Here's how the part is built. I have some questions about the finished solid (model axes, mm). A direction names the side the tool comes from. Coordinates: 2 decimals unless noted, no trailing zeros. Loops run counter-clockwise (first coordinate to the right, second up) from the corner with the lowest first, then second, coordinate; pieces in that order, holes last. Notation, with made-up numbers: M 5.25,-30 L 10.25,-30 A30 ccw 10.25,5 Z; hole C -4.75,11 d6. An arc over 180 degrees is marked long. Use one line per item in the form item = value. Start each with the question number.
(1) Imagine slicing it at B-B, the plane y = -17.5. Please give me the cut outline in (x, z), and give its area (3 significant figures).
(2) On a 3-axis mill with a long thin cutter (end or side, diameter ignored), from which of +Z, -Z, +X, -X, +Y, -Y can I reach the whole of each face in a straight line? I mean faces 1 (the flat face through (9.329, -13, -61)), 2 (the flat face through (-6.824, -22.824, 1.791)), 3 (the flat face through (-14, -13, -46.523)). Say none if no direction works.
(3) Please list where these lines run through material, in increasing order: L1, parallel to Z at x = 16, y = -7; L2, parallel to X at y = -13, z = 27; L3, parallel to Y at x = 6, z = 38.5.
(4) Will these pins go through, and if not, where does the flat tip stop? P1, Ø12, axis at y = -10.5, z = 6, coming from the +X side; P2, Ø10, axis at x = -10.5, y = -22.5, coming from the +Z side; P3, Ø12, axis at y = -14.5, z = 4.5, coming from the -X side; P4, Ø10, axis at x = 13, y = -15, coming from the -Z side.
(5) Imagine slicing it at C-C, the plane x = 11. Please give me the cut outline in (y, z).
(6) Imagine slicing it at D-D, the plane x = -6.5. Please give me the cut outline in (y, z), and give its area (3 significant figures).
(7) Imagine slicing it at A-A, the plane z = -7. Please give me the cut outline in (x, y), and give its area (3 significant figures).
```python
from build123d import *

# Parameters (mm, degrees)
F0_W        = 9.0893283486
F0_H        = 21.5273555368
F0_W_2      = 9.3285199255
F0_H_2      = 29.4207185507
F1_DEPTH    = 25.4
F2_R        = 9.5587418967
F3_DEPTH    = 25.4
F4_C1_SIZE  = 5.08
F4_C2_SIZE  = 5.08
F4_C3_SIZE  = 5.08
F4_C4_SIZE  = 5.08
F4_C5_SIZE  = 5.08
F4_C6_SIZE  = 5.0799
F4_C7_SIZE  = 5.08
F4_C8_SIZE  = 5.08
F4_C9_SIZE  = 5.08
F4_C10_SIZE = 5.08
F4_C11_SIZE = 5.08
F4_C12_SIZE = 5.08
F5_C1_SIZE  = 5.08
F5_C2_SIZE  = 5.08
F5_C3_SIZE  = 5.08
F5_C4_SIZE  = 5.08
F5_C5_SIZE  = 5.08
F5_C6_SIZE  = 5.08
F5_C7_SIZE  = 5.08
F5_C8_SIZE  = 5.08
F5_C9_SIZE  = 5.08
F5_C10_SIZE = 5.08
F5_C11_SIZE = 5.0799
F5_C12_SIZE = 5.08


# Not quite as in the source:
# - a fillet or chamfer is up to 0.001 mm smaller than in the source, because OpenCascade refuses the exact size


with BuildPart() as f1:
    # F0 (on Front) → F1 (new body)
    with BuildSketch(Plane.XZ):
        with Locations((-13.8731840998, -35.7593270019)):
            Rectangle(F0_W, F0_H)
        Polygon((-9.3285199255, -24.9956492335), (-9.3285199255, -46.5230047703), (0, -46.5230047703), (9.3285199255, -46.5230047703), (9.3285199255, -24.9956492335), (9.3285199255, 34.5633625984), (9.3285199255, 71.3990554214), (6.6973981448, 68.2895556092), (-9.3285199255, 34.5633625984), align=None)
        with Locations((13.8731840998, -35.7593270019)):
            Rectangle(F0_W, F0_H)
        with Locations((-4.6642599627, -61.2333640456)):
            Rectangle(F0_W_2, F0_H_2)
        with Locations((4.6642599627, -61.2333640456)):
            Rectangle(F0_W_2, F0_H_2)
    extrude(amount=F1_DEPTH)

    # F2 (on Front) → F3 (join)
    with BuildSketch(Plane.XZ):
        with Locations((0, -37.1944867074)):
            Circle(F2_R)
    extrude(amount=F3_DEPTH)

    # F4: chamfer of 5.08 on 13 edges, made by hand

    # F4_c1
    f4_c1_edges = [f1.edges().sort_by_distance(p)[0] for p in [
        (-13.8731840998, 0, -46.5230047703),
    ]]
    chamfer(f4_c1_edges, length=F4_C1_SIZE)

    # F4_c2
    f4_c2_edges = [f1.edges().sort_by_distance(p)[0] for p in [
        (-18.4178482741, 0, -33.2193270019),
    ]]
    chamfer(f4_c2_edges, length=F4_C2_SIZE)

    # F4_c3
    f4_c3_edges = [f1.edges().sort_by_distance(p)[0] for p in [
        (-9.3285199255, 0, -61.2333640456),
    ]]
    chamfer(f4_c3_edges, length=F4_C3_SIZE)

    # F4_c4
    f4_c4_edges = [f1.edges().sort_by_distance(p)[0] for p in [
        (2.54, 0, -75.943723321),
    ]]
    chamfer(f4_c4_edges, length=F4_C4_SIZE)

    # F4_c5
    f4_c5_edges = [f1.edges().sort_by_distance(p)[0] for p in [
        (9.3285199255, 0, -58.6933640456),
    ]]
    chamfer(f4_c5_edges, length=F4_C5_SIZE)

    # F4_c6 (size 5.08 in the source; OpenCascade refuses exactly that, so slightly less here)
    f4_c6_edges = [f1.edges().sort_by_distance(p)[0] for p in [
        (13.8731840998, 0, -46.5230047703),
    ]]
    chamfer(f4_c6_edges, length=F4_C6_SIZE)

    # F4_c7
    f4_c7_edges = [f1.edges().sort_by_distance(p)[0] for p in [
        (18.4178482741, 0, -33.2193770019),
    ]]
    chamfer(f4_c7_edges, length=F4_C7_SIZE)

    # F4_c8
    f4_c8_edges = [f1.edges().sort_by_distance(p)[0] for p in [
        (11.3331840998, 0, -24.9956492335),
    ]]
    chamfer(f4_c8_edges, length=F4_C8_SIZE)

    # F4_c9
    f4_c9_edges = [f1.edges().sort_by_distance(p)[0] for p in [
        (9.3285199255, 0, 23.2017030939),
    ]]
    chamfer(f4_c9_edges, length=F4_C9_SIZE)

    # F4_c10
    f4_c10_edges = [f1.edges().sort_by_distance(p)[0] for p in [
        (-2.54, 0, 48.8496538587),
    ]]
    chamfer(f4_c10_edges, length=F4_C10_SIZE)

    # F4_c11
    f4_c11_edges = [f1.edges().sort_by_distance(p)[0] for p in [
        (-9.3285199255, 0, -1.1343040268),
    ]]
    chamfer(f4_c11_edges, length=F4_C11_SIZE)

    # F4_c12
    f4_c12_edges = [f1.edges().sort_by_distance(p)[0] for p in [
        (-11.3331840998, 0, -24.9956492335),
    ]]
    chamfer(f4_c12_edges, length=F4_C12_SIZE)

    # F5: chamfer of 5.08 on 13 edges, made by hand

    # F5_c1
    f5_c1_edges = [f1.edges().sort_by_distance(p)[0] for p in [
        (-18.4178482741, -25.4, -35.7593270019),
    ]]
    chamfer(f5_c1_edges, length=F5_C1_SIZE)

    # F5_c2
    f5_c2_edges = [f1.edges().sort_by_distance(p)[0] for p in [
        (-11.3331840998, -25.4, -24.9956492335),
    ]]
    chamfer(f5_c2_edges, length=F5_C2_SIZE)

    # F5_c3
    f5_c3_edges = [f1.edges().sort_by_distance(p)[0] for p in [
        (-11.3331840998, -25.4, -46.5230047703),
    ]]
    chamfer(f5_c3_edges, length=F5_C3_SIZE)

    # F5_c4
    f5_c4_edges = [f1.edges().sort_by_distance(p)[0] for p in [
        (-9.3285199255, -25.4, 4.7838566825),
    ]]
    chamfer(f5_c4_edges, length=F5_C4_SIZE)

    # F5_c5
    f5_c5_edges = [f1.edges().sort_by_distance(p)[0] for p in [
        (-9.3285199255, -25.4, -61.2333640456),
    ]]
    chamfer(f5_c5_edges, length=F5_C5_SIZE)

    # F5_c6
    f5_c6_edges = [f1.edges().sort_by_distance(p)[0] for p in [
        (1.2244391096, -25.4, 56.7718333827),
    ]]
    chamfer(f5_c6_edges, length=F5_C6_SIZE)

    # F5_c7
    f5_c7_edges = [f1.edges().sort_by_distance(p)[0] for p in [
        (2.54, -25.4, -75.943723321),
    ]]
    chamfer(f5_c7_edges, length=F5_C7_SIZE)

    # F5_c8
    f5_c8_edges = [f1.edges().sort_by_distance(p)[0] for p in [
        (9.3285199255, -25.4, 18.4973615123),
    ]]
    chamfer(f5_c8_edges, length=F5_C8_SIZE)

    # F5_c9
    f5_c9_edges = [f1.edges().sort_by_distance(p)[0] for p in [
        (13.8731840998, -25.4, -46.5230047703),
    ]]
    chamfer(f5_c9_edges, length=F5_C9_SIZE)

    # F5_c10
    f5_c10_edges = [f1.edges().sort_by_distance(p)[0] for p in [
        (9.3285199255, -25.4, -58.6933640456),
    ]]
    chamfer(f5_c10_edges, length=F5_C10_SIZE)

    # F5_c11 (size 5.08 in the source; OpenCascade refuses exactly that, so slightly less here)
    f5_c11_edges = [f1.edges().sort_by_distance(p)[0] for p in [
        (13.8731840998, -25.4, -24.9956492335),
    ]]
    chamfer(f5_c11_edges, length=F5_C11_SIZE)

    # F5_c12
    f5_c12_edges = [f1.edges().sort_by_distance(p)[0] for p in [
        (18.4178482741, -25.4, -35.7592770019),
    ]]
    chamfer(f5_c12_edges, length=F5_C12_SIZE)


solid = f1.part
```
Answer:
q1.outline = M -18.42,-46.52 L -9.33,-46.52 L -9.33,-75.94 L 9.33,-75.94 L 9.33,-46.52 L 18.42,-46.52 L 18.42,-25 L 9.33,-25 L 9.33,71.4 L 6.7,68.29 L -9.33,34.56 L -9.33,-25 L -18.42,-25 Z
q1.area = 2,820 mm²
q2.face_1 = -Z, +X, +Y, -Y
q2.face_2 = +Z, -X, -Y
q2.face_3 = -Z, -X, +Y, -Y
q3.L1 = -46.52 to -25
q3.L2 = -9.33 to 9.33
q3.L3 = -23.65 to -1.75
q4.P1 = 9.33
q4.P2 = 41.57
q4.P3 = -9.33
q4.P4 = -75.94
q5.outline = M -25.4,-41.44 L -20.32,-46.52 L -5.08,-46.52 L 0,-41.44 L 0,-30.08 L -5.08,-25 L -20.32,-25 L -25.4,-30.08 Z
q6.outline = M -25.4,-41.44 L -23.15,-43.69 L -23.15,-73.12 L -20.32,-75.94 L -5.08,-75.94 L -2.25,-73.12 L -2.25,-43.69 L 0,-41.44 L 0,-30.08 L -2.25,-27.82 L -2.25,33.93 L -5.08,40.52 L -20.32,40.52 L -23.15,33.93 L -23.15,-27.82 L -25.4,-30.08 Z
q6.area = 2,470 mm²
q7.outline = M -9.33,-20.32 L -4.25,-25.4 L 4.25,-25.4 L 9.33,-20.32 L 9.33,-5.08 L 4.25,0 L -4.25,0 L -9.33,-5.08 Z
q7.area = 422 mm²
